Verification items for this drawing (mm, ordinates from the low corner). A direction names the side the tool comes from. Give positions to 0.01 mm unless a question says otherwise; leave off trailing zeros. Loops run counter-clockwise (first coordinate to the right, second up) from the corner with the lowest first, then second, coordinate; pieces in that order, holes last. Notation, with made-up numbers: M -15.75,79.5 L -4.75,79.5 A15 cw -4.75,103.5 Z; hole C 15.5,58.25 d9. An arc over 180 degrees is marked long. Write each question's results on one line, items separated by ' | '. Start each with the question number.
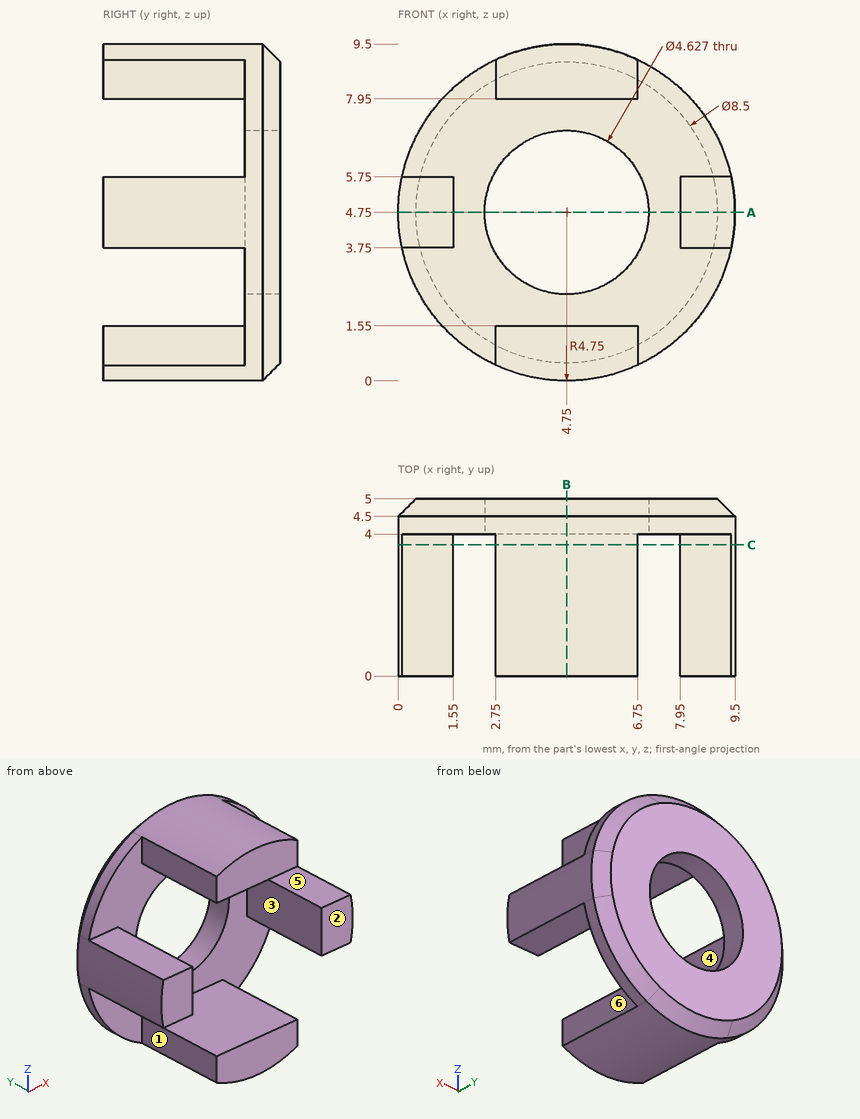
1. Set-up check for the marked faces 4, 5 and 6: record each of +Z, -Z, +X, -X, +Y, -Y from which the full face is reachable in a straight line by a thin tool's end or side.
2. Depth check by flat-ended pin: pin 1 Ø2 at (x, y) = (4.5, 1.5) entering from -Z; pin 2 Ø1.6 at (x, y) = (8.5, 1) entering from -Z; pin 3 Ø3 at (x, y) = (7.5, 1.5) entering from -Z; pin 4 Ø1.2 at (y, z) = (3, 8.5) entering from -X. Enter the tip coordinate at first touch or a pass-through.
3. Release check for a two-part mould opening along X. For the marked faces 1, 2 and 3 record: released by +X, released by -X, zero draft, split by the parting line, or undercut.
4. Thickness scan on probe 1 along X at (y, z) = (4.3, 4.75); probe 2 along Z at (x, y) = (8.5, 2.75); probe 3 along Z at (x, y) = (5.25, 0.65). Record the ranges inside material, lowest first.
5. Section check B-B, the plane x = 4.75. Record the boundary of the cut face in (y, z).
6. Section check A-A, the plane z = 4.75. Record the boundary of the cut face in (x, y), plus the area to 3 significant figures.
7. Section check C-C, the plane y = 3.7. Record the boundary of the cut face in (x, z), plus the area to 3 significant figures.
Filled sheet:
1) face 4: +Z, -Z, -Y | face 5: +Z, +X, -X, -Y | face 6: +Z, -Z, +X, -Y
2) pin 1: z = 0 | pin 2: z = 3.75 | pin 3: z = 0.17 | pin 4: x = 2.75
3) face 1: released by -X | face 2: zero draft | face 3: undercut
4) probe 1: 0 to 2.44, 7.06 to 9.5 | probe 2: 3.75 to 5.75 | probe 3: 0.03 to 1.55, 7.95 to 9.47
5) outline: M 0,0 L 4.5,0 L 5,0.5 L 5,2.44 L 4,2.44 L 4,1.55 L 0,1.55 Z; M 0,7.95 L 4,7.95 L 4,7.06 L 5,7.06 L 5,9 L 4.5,9.5 L 0,9.5 Z
6) outline: M 0,0 L 1.55,0 L 1.55,4 L 2.44,4 L 2.44,5 L 0.5,5 L 0,4.5 Z; M 7.06,4 L 7.95,4 L 7.95,0 L 9.5,0 L 9.5,4.5 L 9,5 L 7.06,5 Z | area: 17.0 mm2
7) outline: M 0.11,3.75 L 1.55,3.75 L 1.55,5.75 L 0.11,5.75 A4.75 ccw Z; M 2.75,0.44 A4.75 ccw 6.75,0.44 L 6.75,1.55 L 2.75,1.55 Z; M 2.75,7.95 L 6.75,7.95 L 6.75,9.06 A4.75 ccw 2.75,9.06 Z; M 7.95,3.75 L 9.39,3.75 A4.75 ccw 9.39,5.75 L 7.95,5.75 Z | area: 17.3 mm2
